```python
from build123d import *

# Parameters (mm, degrees)
BASE_FLANGE3_DEPTH  = 6
SKETCH14_W          = 0.2
SKETCH14_H          = 1
CUT_EXTRUDE1_DEPTH  = 10.97196069
SKETCH15_W          = 2.2
SKETCH15_H          = 2.2
BOSS_EXTRUDE1_DEPTH = 0.5
SKETCH16_W          = 3
SKETCH16_H          = 4.2
BOSS_EXTRUDE2_DEPTH = 0.5


# Sheet-metal steps are written as plain solids
with BuildPart() as part:
    # Sketch1 → Base-Flange3 (new body)
    with BuildSketch(Plane(origin=(0, 0, 0), x_dir=(1, 0, 0), z_dir=(0, 1, 0))):
        with BuildLine():
            Line((6.9, 3), (6.9, 0.1))
            ThreePointArc((6.9, 0.1), (6.870710678, 0.029289322), (6.8, 0))
            Line((6.8, 0), (0.1, 0))
            ThreePointArc((0.1, 0), (0.029289322, 0.029289322), (0, 0.1))
            Line((0, 0.1), (0, 3.7))
            Line((0, 3.7), (-0.1, 3.7))
            Line((-0.1, 3.7), (-0.1, 0.1))
            ThreePointArc((-0.1, 0.1), (-0.041421356, -0.041421356), (0.1, -0.1))
            Line((0.1, -0.1), (6.8, -0.1))
            ThreePointArc((6.8, -0.1), (6.941421356, -0.041421356), (7, 0.1))
            Line((7, 0.1), (7, 3))
            Line((7, 3), (6.9, 3))
        make_face()
    extrude(amount=BASE_FLANGE3_DEPTH)

    # Sketch14 → Cut-Extrude1 (cut, through all)
    with BuildSketch(Plane.XY.offset(0.1)):
        with Locations((0, 0.5)):
            Rectangle(SKETCH14_W, SKETCH14_H)
        with Locations((6.9, 0.5)):
            Rectangle(SKETCH14_W, SKETCH14_H)
    extrude(amount=-CUT_EXTRUDE1_DEPTH, mode=Mode.SUBTRACT)

    # Sketch15 → Boss-Extrude1 (add)
    with BuildSketch(Plane.XY.offset(0.1)):
        with Locations((1.369926131, 2.6)):
            Rectangle(SKETCH15_W, SKETCH15_H)
    extrude(amount=BOSS_EXTRUDE1_DEPTH)

    # Sketch16 → Boss-Extrude2 (add)
    with BuildSketch(Plane.ZY.offset(0.1)):
        with Locations((-2, 3.160264221)):
            Rectangle(SKETCH16_W, SKETCH16_H)
    extrude(amount=BOSS_EXTRUDE2_DEPTH)


solid = part.part
```
The model under review builds one solid part; all positions refer to its coordinate system, in mm. Round coordinates to 2 decimals unless told otherwise and drop trailing zeros. Loops run counter-clockwise (first coordinate to the right, second up) from the corner with the lowest first, then second, coordinate; pieces in that order, holes last.
1) Consider section D-D on y = 2.55. State the section outline as (x, z) points.
Values follow:
outline: (-0.6, -3.5) - (-0.1, -3.5) - (-0.1, -3.7) - (0, -3.7) - (0, -0.1) arc R0.1 cw to (0.1, 0) - (6.8, 0) arc R0.1 cw to (6.9, -0.1) - (6.9, -3) - (7, -3) - (7, -0.1) arc R0.2 ccw to (6.8, 0.1) - (2.47, 0.1) - (2.47, 0.6) - (0.27, 0.6) - (0.27, 0.1) - (0.1, 0.1) arc R0.2 ccw to (-0.1, -0.1) - (-0.1, -0.5) - (-0.6, -0.5) - close
2) Consider section B-B on y = 5.5. State the section outline as (x, z) points.
Values follow:
outline: (-0.1, -3.7) - (0, -3.7) - (0, -0.1) arc R0.1 cw to (0.1, 0) - (6.8, 0) arc R0.1 cw to (6.9, -0.1) - (6.9, -3) - (7, -3) - (7, -0.1) arc R0.2 ccw to (6.8, 0.1) - (0.1, 0.1) arc R0.2 ccw to (-0.1, -0.1) - close
3) Wall thickness on line 1 along Z through (x, y) = (1, 3.55); line 2 along X through (y, z) = (3.45, 0.3): over which ranges is each line inside the solid? List them lowest first.
Values follow:
line 1: z = 0 to 0.6
line 2: x = 0.27 to 2.47
4) Clearance check with flat-ended pins moving along their axes: P1, Ø3, axis at x = 3, y = 3, coming from the -Z side; P2, Ø1.5, axis at x = 5, z = -2, coming from the -Y side; P3, Ø0.6, axis at x = -0.5, y = 4, coming from the -Z side. State where each tip first meets the part, or that it passes through.
Values follow:
P1: stops at z = 0
P2: passes through
P3: stops at z = -3.5
5) Consider section C-C on x = 1.5. State the section outline as (y, z) points, then the cut area to 3 significant figures.
Values follow:
outline: (0, 0) - (6, 0) - (6, 0.1) - (3.7, 0.1) - (3.7, 0.6) - (1.5, 0.6) - (1.5, 0.1) - (0, 0.1) - close
area: 1.70 mm2
6) The part is to be moulded in two halves that separate along X. For faces 1 (the face through (1, 3, 0.6)), 2 (the face through (0, 3, -2)), 3 (the face through (-0.6, 3, -2)), say which applies: pulls with the +X half, pulls with the -X half, needs draft (parallel to the pull), parting line crosses it, or undercut.
Values follow:
face 1: needs draft
face 2: undercut
face 3: pulls with the -X half
7) Consider section A-A on z = -0.7. State the section outline as (x, y) points.
Values follow:
outline: (-0.6, 1.06) - (-0.1, 1.06) - (-0.1, 1) - (0, 1) - (0, 6) - (-0.1, 6) - (-0.1, 5.26) - (-0.6, 5.26) - close; (6.9, 1) - (7, 1) - (7, 6) - (6.9, 6) - close
